```python
from build123d import *

# Parameters (mm, degrees)
PAD_DEPTH    = 15
SKETCH001_R  = 1.6
POCKET_DEPTH = 10.001
CHAMFER_SIZE = 1


with BuildPart() as part:
    # Sketch → Pad (new body)
    with BuildSketch(Plane.XY):
        with BuildLine():
            ThreePointArc((-2, 3), (-6, 7), (-10, 3))
            Line((-10, 3), (-10, 0))
            Line((-10, 0), (-15, 0))
            Line((-15, 0), (-15, 10))
            Line((15, 10), (-15, 10))
            Line((15, 0), (15, 10))
            Line((10, 0), (15, 0))
            Line((10, 3), (10, 0))
            ThreePointArc((10, 3), (6, 7), (2, 3))
            Line((2, 0), (2, 3))
            Line((-2, 0), (2, 0))
            Line((-2, 3), (-2, 0))
        make_face()
    extrude(amount=PAD_DEPTH)

    # Sketch001 → Pocket (cut, through all)
    with BuildSketch(Plane.XZ):
        with Locations((0, 7.5)):
            Circle(SKETCH001_R)
        with Locations((-12, 7.5)):
            Circle(SKETCH001_R)
        with Locations((12, 7.5)):
            Circle(SKETCH001_R)
    extrude(amount=-POCKET_DEPTH, mode=Mode.SUBTRACT)

    # Chamfer
    chamfer_edges = [part.edges().sort_by_distance(p)[0] for p in [
        (-2, 1.5, 15),
        (-6, 7, 15),
        (-10, 1.5, 15),
        (-12.5, 0, 15),
        (-15, 5, 15),
        (0, 10, 15),
        (15, 5, 15),
        (12.5, 0, 15),
        (10, 1.5, 15),
        (6, 7, 15),
        (2, 1.5, 15),
        (0, 0, 15),
        (-2, 1.5, 0),
        (-6, 7, 0),
        (-10, 1.5, 0),
        (-12.5, 0, 0),
        (-15, 5, 0),
        (0, 10, 0),
        (15, 5, 0),
        (12.5, 0, 0),
        (10, 1.5, 0),
        (6, 7, 0),
        (2, 1.5, 0),
        (0, 0, 0),
    ]]
    chamfer(chamfer_edges, length=CHAMFER_SIZE)


solid = part.part
```
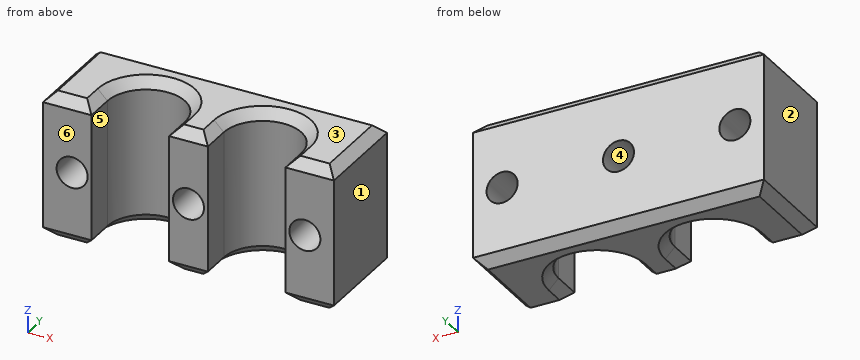
Source: CAD feature listing. Evaluate the final solid. Frame: model axes, mm. Face numbers are marked on the shaded views. A direction names the side the tool comes from. Give positions to 0.01 mm unless a question says otherwise; leave off trailing zeros. Loops run counter-clockwise (first coordinate to the right, second up) from the corner with the lowest first, then second, coordinate; pieces in that order, holes last. Notation, with made-up numbers: (52, 61.5) -> (67, 61.5) arc R13 ccw to (67, 83.5) -> close; hole circle Ø2 at (72, 17). An arc over 180 degrees is marked (long way). Put each result on its own line as item: value. Start each with the question number.
1) Draft query along X for the marked faces 1, 2, 3 and 4. Return one class per face: released by +X, released by -X, zero draft, split by the parting line, or undercut.
2) Material intervals for probe 1 along Z at (x, y) = (0, 4.75); probe 2 along X at (y, z) = (4.75, 12.75); probe 3 along X at (y, z) = (5, 6.25), sorted ascending.
3) Cut plane D-D (z = 8.5). Return loops of the section in (x, y).
4) Contact query for flat-ended pins moving along their axis: P1, Ø1.5, axis at x = -8, y = 6.5, coming from the -Z side; P2, Ø3, axis at x = -12, z = 7.5, coming from the +Y side. Output: stop coordinate, or through.
5) Cut plane B-B (z = 4.75). Return loops of the section in (x, y).
6) Reachability of the marked faces 5 and 6 from +Z, -Z, +X, -X, +Y, -Y: full face, straight path, thin tool, end or side. Return the list, or none.
7) Cut plane C-C (x = -6). Return loops of the section in (y, z).
8) Cut plane A-A (x = 12). Return loops of the section in (y, z).
Results are:
1. face 1: released by +X
1. face 2: released by -X
1. face 3: zero draft
1. face 4: undercut
2. probe 1: z = 0 to 5.9, 9.1 to 15
2. probe 2: x = -15 to -9.6, -2.4 to 2.4, 9.6 to 15
2. probe 3: x = -15 to -13, -11 to -9.46, -2.54 to -1, 1 to 2.54, 9.46 to 11, 13 to 15
3. outline: (-15, 0) -> (-13.25, 0) -> (-13.25, 10) -> (-15, 10) -> close; (-10.75, 0) -> (-10, 0) -> (-10, 3) arc R4 cw to (-2, 3) -> (-2, 0) -> (-1.25, 0) -> (-1.25, 10) -> (-10.75, 10) -> close; (1.25, 0) -> (2, 0) -> (2, 3) arc R4 cw to (10, 3) -> (10, 0) -> (10.75, 0) -> (10.75, 10) -> (1.25, 10) -> close; (13.25, 0) -> (15, 0) -> (15, 10) -> (13.25, 10) -> close
4. P1: stops at z = 0.22
4. P2: passes through
5. outline: (-15, 0) -> (-10, 0) -> (-10, 3) arc R4 cw to (-2, 3) -> (-2, 0) -> (2, 0) -> (2, 3) arc R4 cw to (10, 3) -> (10, 0) -> (15, 0) -> (15, 10) -> (-15, 10) -> close
6. face 5: +Z, -Z, -Y
6. face 6: +Z, -Z, +X, -X, -Y
7. outline: (7, 1) -> (8, 0) -> (9, 0) -> (10, 1) -> (10, 14) -> (9, 15) -> (8, 15) -> (7, 14) -> close
8. outline: (0, 1) -> (1, 0) -> (9, 0) -> (10, 1) -> (10, 5.9) -> (0, 5.9) -> close; (0, 9.1) -> (10, 9.1) -> (10, 14) -> (9, 15) -> (1, 15) -> (0, 14) -> close
